Geometry check sheet. Reference: the model listing, model coordinates, mm. Face numbers are marked on the shaded views. A direction names the side the tool comes from. Round coordinates to 2 decimals unless told otherwise and drop trailing zeros. Write each loop counter-clockwise with the first axis right and the second up, starting at its lowest first coordinate (ties: lowest second). Pieces come first, ordered by that corner, then holes. Notation, with made-up numbers: M 32.25,-40 L 78.25,-40 A29 cw 78.25,-11 Z; hole C 67.25,65 d6. An arc over 180 degrees is marked long. One line per item, written item: value. Start each with the question number.
1. Section check A-A (x = 0). Record the boundary of the cut face in (y, z) (3 decimals), and give its area (3 significant figures).
2. Section check D-D (z = -0.5). Record the boundary of the cut face in (x, y).
3. Release check for a two-part mould opening along Y. For the marked faces 3, 4 and 5 record: pulls with the +Y half, pulls with the -Y half, needs draft (parallel to the pull), parting line crosses it, or undercut.
4. Section check C-C (z = 1). Record the boundary of the cut face in (x, y), and give its area (3 significant figures).
5. Depth check by flat-ended pin: P1, Ø2, axis at y = 3.5, z = 2, coming from the +X side; P2, Ø1.5, axis at y = 0, z = 1.5, coming from the -X side; P3, Ø3, axis at x = 9, z = -0.5, coming from the -Y side. Enter the tip coordinate at first touch or a pass-through.
6. Scan lines: probe 1 along Y at (x, z) = (0, 1.45); probe 2 along Z at (x, y) = (9.5, -1); probe 3 along X at (y, z) = (-6, -1.25). Record each from-to range of solid material in increasing order. Write a range as [from, to].
7. Access from +Z, -Z, +X, -X, +Y, -Y to the whole of each face (thin tool, end or side, straight path). Record for the marked faces 1 and 2.
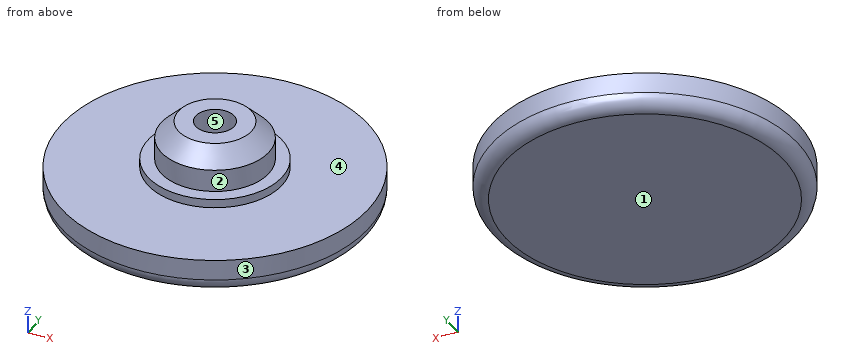
from build123d import *

# Parameters (mm, degrees)
F0_R     = 3.95
F1_DEPTH = 3.556
F0_R_2   = 11.2522
F2_DEPTH = 2.54
F3_R     = 1.016
F4_R     = 4.9244336153
F4_R_2   = 3.95
F5_DEPTH = 0.635
F6_T     = -2.54
F7_SIZE  = 1.27


with BuildPart() as f1:
    # F0 (on Top) → F1 (new body)
    with BuildSketch(Plane.XY):
        Circle(F0_R)
    extrude(amount=F1_DEPTH)

    # F0 (on Top) → F2 (join)
    with BuildSketch(Plane.XY):
        Circle(F0_R_2)
        Circle(F0_R, mode=Mode.SUBTRACT)
        Circle(F0_R)
    extrude(amount=-F2_DEPTH)

    # F3
    f3_edges = [f1.edges().sort_by_distance(p)[0] for p in [
        (-11.2522, 0, -2.54),
    ]]
    fillet(f3_edges, radius=F3_R)

    # F4 (on face) → F5 (join, symmetric)
    with BuildSketch(Plane.XY):
        Circle(F4_R)
        Circle(F4_R_2, mode=Mode.SUBTRACT)
    extrude(amount=F5_DEPTH, both=True)

    # F6
    f6_openings = [f1.faces().sort_by_distance(p)[0] for p in [
        (0, 0, 3.556),
    ]]
    offset(amount=F6_T, openings=f6_openings, kind=Kind.INTERSECTION)

    # F7
    f7_edges = [f1.edges().sort_by_distance(p)[0] for p in [
        (-3.95, 0, 3.556),
    ]]
    chamfer(f7_edges, length=F7_SIZE)


solid = f1.part
Result sheet:
1. outline: M -11.252,-1.524 A1.016 ccw -10.236,-2.54 L 10.236,-2.54 A1.016 ccw 11.252,-1.524 L 11.252,0 L 4.924,0 L 4.924,0.635 L 3.95,0.635 L 3.95,2.286 L 2.68,3.556 L 1.41,3.556 L 1.41,0 L -1.41,0 L -1.41,3.556 L -2.68,3.556 L -3.95,2.286 L -3.95,0.635 L -4.924,0.635 L -4.924,0 L -11.252,0 Z
1. area: 74.4 mm2
2. outline: C 0,0 d22.5
3. face 3: parting line crosses it
3. face 4: needs draft
3. face 5: undercut
4. outline: C 0,0 d7.9; hole C 0,0 d2.82
4. area: 42.8 mm2
5. P1: stops at x = 3.06
5. P2: stops at x = -3.95
5. P3: stops at y = -8.39
6. probe 1: y = [-3.95, -1.41], [1.41, 3.95]
6. probe 2: z = [-2.54, 0]
6. probe 3: x = [-9.52, 9.52]
7. face 1: -Z, +X, -X, +Y, -Y
7. face 2: +Z
